The listing builds one solid part. Answer for the finished solid, in the listing's coordinates (mm). Face numbers are marked on the shaded views. A direction names the side the tool comes from. Give positions to 0.01 mm unless a question says otherwise; leave off trailing zeros. Loops run counter-clockwise (first coordinate to the right, second up) from the corner with the lowest first, then second, coordinate; pieces in that order, holes last. Notation, with made-up numbers: (21, 78) - (45, 78) arc R8 cw to (45, 90) - close; hole circle Ø1 at (-1.5, 10). An arc over 180 degrees is marked (long way). Write each question's results on one line, items separated by ' | '.
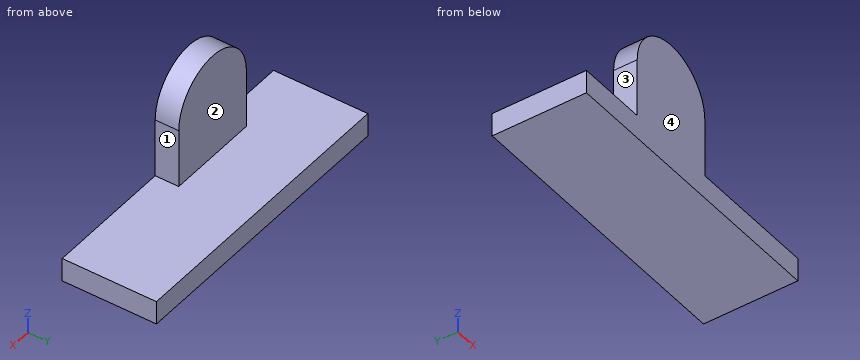
from build123d import *

# Parameters (mm, degrees)
F0_W     = 125
F0_H     = 40
F1_DEPTH = 10
F3_DEPTH = 10


with BuildPart() as f1:
    # F0 (on Top) → F1 (new body)
    with BuildSketch(Plane.XY):
        with Locations((62.5, 20)):
            Rectangle(F0_W, F0_H)
    extrude(amount=F1_DEPTH)

    # F2 (on face) → F3 (join)
    with BuildSketch(Plane.XZ):
        with BuildLine():
            Line((30, 35), (30, 0))
            Line((30, 0), (70, 0))
            Line((70, 0), (70, 35))
            ThreePointArc((70, 35), (50, 55), (30, 35))
        make_face()
    extrude(amount=-F3_DEPTH)


solid = f1.part
Item 1: A cutting plane is placed at B-B, the plane x = 50. Determine the outline of the cut face in (y, z), plus the area to 3 significant figures.
Values found:
outline: (0, 0) - (40, 0) - (40, 10) - (10, 10) - (10, 55) - (0, 55) - close | area: 850 mm²
Item 2: Flat-ended cylindrical pins translate along their axes: P1, Ø6, axis at x = 33, y = 5, coming from the +Z side; P2, Ø8, axis at y = 3.5, z = 25.5, coming from the +X side; P3, Ø6, axis at x = 75, y = 24.5, coming from the +Z side. Find the tip coordinate at first contact, or state that the pin passes through.
Values found:
P1: stops at z = 49.28 | P2: stops at x = 70 | P3: stops at z = 10
Item 3: A cutting plane is placed at C-C, the plane z = 33. Determine the outline of the cut face in (x, y).
Values found:
outline: (30, 0) - (70, 0) - (70, 10) - (30, 10) - close
Item 4: A cutting plane is placed at A-A, the plane y = 4. Determine the outline of the cut face in (x, z), plus the area to 3 significant figures.
Values found:
outline: (0, 0) - (125, 0) - (125, 10) - (70, 10) - (70, 35) arc R20 ccw to (30, 35) - (30, 10) - (0, 10) - close | area: 2,880 mm²
Item 5: Find the intervals of material crossed by line 1 along Y through (x, z) = (36, 41.5); line 2 along X through (y, z) = (4, 30.5), in increasing order. Write a range as [from, to].
Values found:
line 1: y = [0, 10] | line 2: x = [30, 70]
Item 6: A cutting plane is placed at D-D, the plane y = 23.5. Determine the outline of the cut face in (x, z).
Values found:
outline: (0, 0) - (125, 0) - (125, 10) - (0, 10) - close
Item 7: For the marked faces 1, 2, 3 and 4, determine the directions among +Z, -Z, +X, -X, +Y, -Y from which every point of the face is accessible in a straight line to the end or side of a thin tool.
Values found:
face 1: +Z, +X, +Y, -Y | face 2: +Z, +X, -X, +Y | face 3: +Z, -X, +Y, -Y | face 4: +Z, -Z, +X, -X, -Y
